Here's the drawing with two shaded views (mm, measured from the low corner). I have some questions. Round coordinates to 2 decimals unless told otherwise and drop trailing zeros. Write each loop counter-clockwise with the first axis right and the second up, starting at its lowest first coordinate (ties: lowest second). Pieces come first, ordered by that corner, then holes. Notation, with made-up numbers: M 54.25,-5 L 84.25,-5 A23 cw 84.25,26 Z; hole C 38.25,76 d4. An arc over 180 degrees is marked long. Answer as a JSON object with one key per item and string values. Group by question number.
1) Suppose I cut it at C-C, the plane z = 17.5. Write out the boundary of the cut face in (x, y).
2) Please list where these lines run through material, in increasing order: L1, parallel to Y at x = 46, z = 16; L2, parallel to Y at x = 46, z = 23.25; L3, parallel to Z at x = 10.5, y = 37. Write a range as [from, to].
3) Suppose I cut it at D-D, the plane z = 6. Write out the boundary of the cut face in (x, y), and give its area (3 significant figures).
4) I'm going to push flat-ended pins straight in: pin 1 Ø1 at (x, z) = (49.5, 17) entering from +Y; pin 2 Ø2 at (x, z) = (56, 16) entering from +Y; pin 3 Ø10 at (x, z) = (60.5, 18.5) entering from +Y; pin 4 Ø1.8 at (x, y) = (46, 61.5) entering from -Z. Where does each tip first touch, or does it pass through?
5) Suppose I cut it at A-A, the plane x = 46. Write out the boundary of the cut face in (y, z).
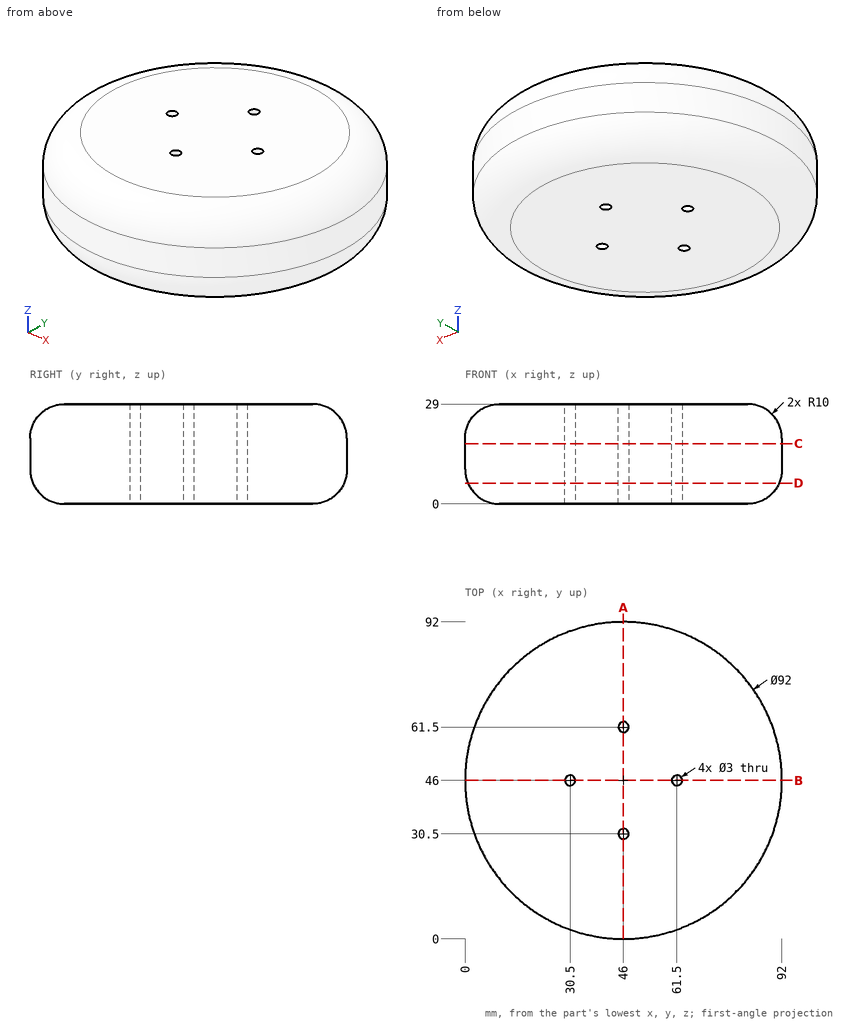
Results:
{
 "1": {"outline": "C 46,46 d92; hole C 30.5,46 d3; hole C 46,30.5 d3; hole C 46,61.5 d3; hole C 61.5,46 d3"},
 "2": {"L1": "[0, 29], [32, 60], [63, 92]", "L2": "[0.95, 29], [32, 60], [63, 91.05]", "L3": "[0.02, 28.98]"},
 "3": {"outline": "C 46,46 d90.33; hole C 30.5,46 d3; hole C 46,30.5 d3; hole C 46,61.5 d3; hole C 61.5,46 d3", "area": "6,380 mm^2"},
 "4": {"pin 1": "y = 91.9", "pin 2": "y = 91.11", "pin 3": "y = 91.01", "pin 4": "through"},
 "5": {"outline": "M 0,10 A10 ccw 10,0 L 29,0 L 29,29 L 10,29 A10 ccw 0,19 Z; M 32,0 L 60,0 L 60,29 L 32,29 Z; M 63,0 L 82,0 A10 ccw 92,10 L 92,19 A10 ccw 82,29 L 63,29 Z"}
}
